```python
from build123d import *

# Parameters (mm, degrees)
BOSS_EXTRUDE1_DEPTH = 19.05
SKETCH2_W           = 11.1125
SKETCH2_H           = 6.604
CUT_EXTRUDE1_DEPTH  = 112.391012889


with BuildPart() as part:
    # Sketch1 → Boss-Extrude1 (new body)
    with BuildSketch(Plane(origin=(0, 0, 0), x_dir=(1, 0, 0), z_dir=(0, 1, 0))):
        with BuildLine():
            Line((0, 6.35), (0, 86.286703653))
            ThreePointArc((0, 86.286703653), (-4.706499064, 92.420332649), (-11.849261314, 89.461703653))
            Line((-11.849261314, 89.461703653), (-58.000738686, 9.525))
            ThreePointArc((-58.000738686, 9.525), (-58.000738686, 3.175), (-52.501477372, 0))
            Line((-52.501477372, 0), (-6.35, 0))
            ThreePointArc((-6.35, 0), (-1.859871939, 1.859871939), (0, 6.35))
        make_face()
    extrude(amount=BOSS_EXTRUDE1_DEPTH)

    # Sketch2 → Cut-Extrude1 (cut, through all)
    with BuildSketch(Plane(origin=(0, 19.05, 0), x_dir=(1, 0, 0), z_dir=(0, 1, 0))):
        with Locations((-29.425738686, 3.302)):
            Rectangle(SKETCH2_W, SKETCH2_H)
    extrude(amount=-CUT_EXTRUDE1_DEPTH, mode=Mode.SUBTRACT)


solid = part.part
```
Build history of the part. All positions in model axes, mm. A direction names the side the tool comes from. Give positions to 0.01 mm unless a question says otherwise; leave off trailing zeros. Order: outer loops, then holes, each group sorted by start corner. A loop starts at its lowest first (then second) coordinate and runs counter-clockwise, first axis right, second up. Notation, with made-up numbers: M 59.5,8 L 73.5,8 A5 cw 73.5,12 Z; hole C 21.5,-36 d2. An arc over 180 degrees is marked long. Write item = value, one per line. Start each with the question number.
(1) Probe L1, parallel to Z at x = -6, y = 17.5; L2, parallel to X at y = 16.5, z = -61.5; L3, parallel to X at y = 12.25, z = -51.5. List the from-to ranges inside material, lowest first. Write a range as [from, to].
(2) Pin check, flat tips, straight feed: pin 1 Ø8 at (x, y) = (-47, 14.5) entering from -Z; pin 2 Ø2 at (y, z) = (13.5, -4) entering from +X; pin 3 Ø1.5 at (x, y) = (-37.5, 3) entering from -Z. Stop position of each tip, or through.
(3) Two-plate mould, pull along X, no slides. Class faces 3 (the flat face through (-23, 0, -37)), 4 (the cylindrical face through (-58.05, 9.39, -3.26)), 5 (the flat face through (-30, 10, -6.604)): released by +X, released by -X, zero draft, split by the parting line, or undercut.
(4) Which spindle directions (+Z, -Z, +X, -X, +Y, -Y) get a long thin tool onto all of the face, cutting with end or side? Do faces 1 (the cylindrical face through (-1.91, 9.39, -1.81)), 2 (the flat face through (-34.982, 10, -3)). Say none if no direction does.
(5) Slice it at A-A on y = 16. Write the cut outline in (x, z) (3 decimals), plus the area to 3 significant figures.
(6) Slice it at B-B on z = -61. Write the cut outline in (x, y).
(7) Slice it at C-C on x = -29.5. Write the cut outline in (y, z), plus the area to 3 significant figures.
Responses:
q1.L1 = [-92.63, -0.01]
q1.L2 = [-27.99, 0]
q1.L3 = [-33.77, 0]
q2.pin_1 = -35.51
q2.pin_2 = -0.15
q2.pin_3 = -46.33
q3.face_3 = zero draft
q3.face_4 = released by -X
q3.face_5 = undercut
q4.face_1 = +Z, +X, +Y, -Y
q4.face_2 = +Z, +Y, -Y
q5.outline = M -58.001,-9.525 L -11.849,-89.462 A6.35 ccw 0,-86.287 L 0,-6.35 A6.35 ccw -6.35,0 L -23.869,0 L -23.869,-6.604 L -34.982,-6.604 L -34.982,0 L -52.501,0 A6.35 ccw Z
q5.area = 3,280 mm2
q6.outline = M -28.28,0 L 0,0 L 0,19.05 L -28.28,19.05 Z
q7.outline = M 0,-58.89 L 19.05,-58.89 L 19.05,-6.6 L 0,-6.6 Z
q7.area = 996 mm2
